Verification items for the finished model (mm, model axes). A direction names the side the tool comes from. Coordinates: 2 decimals unless noted, no trailing zeros. Write each loop counter-clockwise with the first axis right and the second up, starting at its lowest first coordinate (ties: lowest second). Pieces come first, ordered by that corner, then holes. Notation, with made-up numbers: (20, 23) -> (53, 23) arc R12 cw to (53, 30) -> close; hole circle Ø8 at (66.25, 89). An arc over 180 degrees is marked (long way). Answer in a Markdown table with one row per item.
```python
from build123d import *

# Parameters (mm, degrees)
BOSS_EXTRUDE1_DEPTH = 95.25
SKETCH3_W           = 9
SKETCH3_H           = 41.03
CUT_EXTRUDE1_DEPTH  = 183.880891019
SKETCH4_R           = 1.03
CUT_EXTRUDE2_DEPTH  = 3


with BuildPart() as part:
    # Sketch1 → Boss-Extrude1 (new body)
    with BuildSketch(Plane.XY):
        Polygon((0, 0), (0, 18.61), (-165.72, 18.61), (-165.72, -24.03), (-161.52, -24.03), (-161.52, -41.03), (-154.83, -41.03), (-154.83, -24.03), (-150.63, -24.03), (-150.63, 0.01), (-78.94, 0.01), (-78.94, 7.01), (-30.27, 7.01), (-30.27, 0.01), (-13.32, 0.01), (-13.32, 9.54), (-9.63, 9.54), (-9.63, 0), align=None)
    extrude(amount=BOSS_EXTRUDE1_DEPTH)

    # Sketch3 → Cut-Extrude1 (cut, through all)
    with BuildSketch(Plane(origin=(-150.63, 0, 0), x_dir=(0, 0, -1), z_dir=(1, 0, 0))):
        with Locations((-4.5, -20.515)):
            Rectangle(SKETCH3_W, SKETCH3_H)
    extrude(amount=-CUT_EXTRUDE1_DEPTH, mode=Mode.SUBTRACT)

    # Sketch4 → Cut-Extrude2 (cut)
    with BuildSketch(Plane.XZ.offset(-7.01)):
        with Locations(Location((-69.08, 42.44, 0), (0, 0, 270))):
            Circle(SKETCH4_R)
        with Locations(Location((-49.58, 60.2, 0), (0, 0, 270))):
            Circle(SKETCH4_R)
    extrude(amount=-CUT_EXTRUDE2_DEPTH, mode=Mode.SUBTRACT)


solid = part.part
```
1. Access from +Z, -Z, +X, -X, +Y, -Y to the whole of each face (thin tool, end or side, straight path). Record for faces 1 (the face through (-55, 7.01, 47)), 2 (the face through (-158, 0, 5)), 3 (the face through (-154.83, -33, 52)), 4 (the face through (-161.52, -32, 52)).
Findings below:
| item | result |
|---|---|
| face 1 | +Z, -Z, -Y |
| face 2 | -Z, +X, -X, -Y |
| face 3 | +Z, -Z, +X, -Y |
| face 4 | +Z, -Z, -X, -Y |
2. Sectioned sample at C-C, the plane y = -2.5. Record the cut outline in (x, z).
Findings below:
| item | result |
|---|---|
| outline | (-165.72, 9) -> (-150.63, 9) -> (-150.63, 95.25) -> (-165.72, 95.25) -> close |
3. Sectioned sample at B-B, the plane x = -134. Record the cut outline in (y, z), and give its area (3 significant figures).
Findings below:
| item | result |
|---|---|
| outline | (0.01, 0) -> (18.61, 0) -> (18.61, 95.25) -> (0.01, 95.25) -> close |
| area | 1,770 mm² |
4. Sectioned sample at A-A, the plane z = 33. Record the cut outline in (x, y).
Findings below:
| item | result |
|---|---|
| outline | (-165.72, -24.03) -> (-161.52, -24.03) -> (-161.52, -41.03) -> (-154.83, -41.03) -> (-154.83, -24.03) -> (-150.63, -24.03) -> (-150.63, 0.01) -> (-78.94, 0.01) -> (-78.94, 7.01) -> (-30.27, 7.01) -> (-30.27, 0.01) -> (-13.32, 0.01) -> (-13.32, 9.54) -> (-9.63, 9.54) -> (-9.63, 0) -> (0, 0) -> (0, 18.61) -> (-165.72, 18.61) -> close |
5. Material ranges on probe 1 along X at (y, z) = (7.75, 60.2); probe 2 along X at (y, z) = (8.9, 42.44); probe 3 along Z at (x, y) = (-69, 8), recorded low to high. Write a range as from..to.
Findings below:
| item | result |
|---|---|
| probe 1 | x = -165.72..-50.61, -48.55..-13.32, -9.63..0 |
| probe 2 | x = -165.72..-70.11, -68.05..-13.32, -9.63..0 |
| probe 3 | z = 0..41.41, 43.47..95.25 |
6. Go/stop test with flat-tipped pins: pin 1 (13.5 mm diameter, centred on y = -32, z = 67, fed in from -X); pin 2 (10 mm diameter, centred on y = -7.5, z = 57, fed in from +X); pin 3 (4.5 mm diameter, centred on x = -152, z = 58.5, fed in from -Y). Record where each tip stops, or that it passes through.
Findings below:
| item | result |
|---|---|
| pin 1 | stops at x = -161.52 |
| pin 2 | stops at x = -150.63 |
| pin 3 | stops at y = -24.03 |
7. Release check for a two-part mould opening along X. For faces 5 (the face through (-12, 9.54, 47)), 6 (the face through (-82, 18.61, 47)), 7 (the face through (-9.63, 5, 47)), 8 (the face through (-165.72, -2, 47)) record: released by +X, released by -X, zero draft, split by the parting line, or undercut.
Findings below:
| item | result |
|---|---|
| face 5 | undercut |
| face 6 | zero draft |
| face 7 | undercut |
| face 8 | released by -X |
